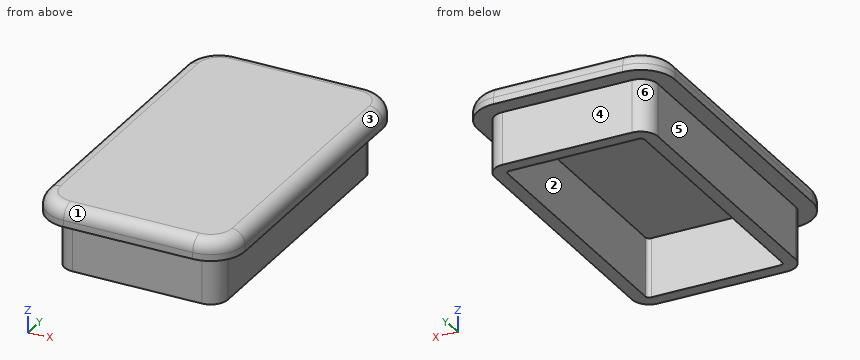
from build123d import *

# Parameters (mm, degrees)
BOSS_EXTRUDE1_DEPTH = 8
BOSS_EXTRUDE3_DEPTH = 3
FILLET1_R           = 2
SHELL1_T            = -2


with BuildPart() as part:
    # Sketch1 → Boss-Extrude1 (new body)
    with BuildSketch(Plane.XY):
        with BuildLine():
            Line((-9.8, -22.4), (9.8, -22.4))
            ThreePointArc((9.8, -22.4), (11.638477631, -21.638477631), (12.4, -19.8))
            Line((12.4, -19.8), (12.4, 19.8))
            ThreePointArc((12.4, 19.8), (11.638477631, 21.638477631), (9.8, 22.4))
            Line((9.8, 22.4), (-9.8, 22.4))
            ThreePointArc((-9.8, 22.4), (-11.638477631, 21.638477631), (-12.4, 19.8))
            Line((-12.4, 19.8), (-12.4, -19.8))
            ThreePointArc((-12.4, -19.8), (-11.638477631, -21.638477631), (-9.8, -22.4))
        make_face()
    extrude(amount=-BOSS_EXTRUDE1_DEPTH)

    # Sketch3 → Boss-Extrude3 (add)
    with BuildSketch(Plane.XY):
        with BuildLine():
            Line((-9.8, -25), (9.8, -25))
            ThreePointArc((9.8, -25), (13.476955262, -23.476955262), (15, -19.8))
            Line((15, -19.8), (15, 19.8))
            ThreePointArc((15, 19.8), (13.476955262, 23.476955262), (9.8, 25))
            Line((9.8, 25), (-9.8, 25))
            ThreePointArc((-9.8, 25), (-13.476955262, 23.476955262), (-15, 19.8))
            Line((-15, 19.8), (-15, -19.8))
            ThreePointArc((-15, -19.8), (-13.476955262, -23.476955262), (-9.8, -25))
        make_face()
    extrude(amount=BOSS_EXTRUDE3_DEPTH)

    # Fillet1
    fillet1_edges = [part.edges().sort_by_distance(p)[0] for p in [
        (13.476955262, 23.476955262, 3),
        (0, 25, 3),
        (-13.476955262, 23.476955262, 3),
        (-15, 0, 3),
        (-13.476955262, -23.476955262, 3),
        (0, -25, 3),
        (13.476955262, -23.476955262, 3),
        (15, 0, 3),
    ]]
    fillet(fillet1_edges, radius=FILLET1_R)

    # Shell1
    shell1_openings = [part.faces().sort_by_distance(p)[0] for p in [
        (0, 0, -8),
    ]]
    offset(amount=SHELL1_T, openings=shell1_openings, kind=Kind.INTERSECTION)


solid = part.part
Model file for the job. Use its own axes, mm. Face numbers are marked on the shaded views. A direction names the side the tool comes from. Round coordinates to 2 decimals unless told otherwise and drop trailing zeros. Loops run counter-clockwise (first coordinate to the right, second up) from the corner with the lowest first, then second, coordinate; pieces in that order, holes last. Notation, with made-up numbers: M 22.25,50.25 L 74.25,50.25 A16 ccw 74.25,77.25 Z; hole C -38.5,58.25 d11. An arc over 180 degrees is marked long. One line per question, with ' | ' between items.
1) Flat gauge pins, fed straight in: pin 1 (6 mm diameter, centred on y = 15, z = -4.5, fed in from -X); pin 2 (2.5 mm diameter, centred on x = 0, z = -5, fed in from -Y); pin 3 (1 mm diameter, centred on x = -3, z = -1, fed in from +Y); pin 4 (6 mm diameter, centred on y = -1.5, z = -2.5, fed in from +X). Where does each tip first touch, or does it go through?
Solved:
pin 1: stops at x = -12.4 | pin 2: stops at y = -22.4 | pin 3: stops at y = 22.4 | pin 4: stops at x = 15
2) Band-saw the part on B-B (z = -4). Give the cut face in (x, y).
Solved:
outline: M -12.4,-19.8 A2.6 ccw -9.8,-22.4 L 9.8,-22.4 A2.6 ccw 12.4,-19.8 L 12.4,19.8 A2.6 ccw 9.8,22.4 L -9.8,22.4 A2.6 ccw -12.4,19.8 Z; hole M -10.4,-19.8 A0.6 ccw -9.8,-20.4 L 9.8,-20.4 A0.6 ccw 10.4,-19.8 L 10.4,19.8 A0.6 ccw 9.8,20.4 L -9.8,20.4 A0.6 ccw -10.4,19.8 Z
3) Drill centre lines: line 1 along Y through (x, z) = (7.5, -5); line 2 along X through (y, z) = (-4, -7.25); line 3 along Y through (x, z) = (6.75, 0.25). Where is each one in solid material? Low to high.
Solved:
line 1: y = -22.4 to -20.4, 20.4 to 22.4 | line 2: x = -12.4 to -10.4, 10.4 to 12.4 | line 3: y = -25 to -20.4, 20.4 to 25
4) Mould opens along X. For the marked faces 1, 2 and 3 say: +X half, -X half, draft (parallel to the pull), parting line (faces both ways), or undercut.
Solved:
face 1: draft | face 2: undercut | face 3: +X half
5) Band-saw the part on C-C (y = 0.5). Give the cut face in (x, z).
Solved:
outline: M -15,0 L -12.4,0 L -12.4,-8 L -10.4,-8 L -10.4,1 L 10.4,1 L 10.4,-8 L 12.4,-8 L 12.4,0 L 15,0 L 15,1 A2 ccw 13,3 L -13,3 A2 ccw -15,1 Z
6) Band-saw the part on A-A (x = -7.5). Give the cut face in (y, z), then the cut area to 3 significant figures.
Solved:
outline: M -25,0 L -22.4,0 L -22.4,-8 L -20.4,-8 L -20.4,1 L 20.4,1 L 20.4,-8 L 22.4,-8 L 22.4,0 L 25,0 L 25,1 A2 ccw 23,3 L -23,3 A2 ccw -25,1 Z | area: 139 mm²
7) 3-axis set-ups, long thin cutter, end or side, ignore diameter. For the marked faces 4, 5 and 6: which of +Z, -Z, +X, -X, +Y, -Y reach the whole face in a straight line?
Solved:
face 4: -Z, +X, -X, +Y | face 5: -Z, -X, +Y, -Y | face 6: -Z, -X, +Y
